```python
from build123d import *

# Parameters (mm, degrees)
SKETCH_R        = 14.1
SKETCH_R_2      = 1
PAD_DEPTH       = 38
SKETCH001_R     = 1.5
POCKET_DEPTH    = 3
SKETCH002_W     = 20
SKETCH002_H     = 2.5
SKETCH002_W_2   = 18
POCKET001_DEPTH = 34.001


with BuildPart() as part:
    # Sketch → Pad (new body)
    with BuildSketch(Plane.XY):
        Polygon((16, -16), (16, 16), (16, 18), (-16, 18), (-16, 16), (-16, -16), align=None)
        Circle(SKETCH_R, mode=Mode.SUBTRACT)
        with Locations((-12, 12)):
            Circle(SKETCH_R_2, mode=Mode.SUBTRACT)
        with Locations((12, 12)):
            Circle(SKETCH_R_2, mode=Mode.SUBTRACT)
        with Locations((12, -12)):
            Circle(SKETCH_R_2, mode=Mode.SUBTRACT)
        with Locations((-12, -12)):
            Circle(SKETCH_R_2, mode=Mode.SUBTRACT)
    extrude(amount=PAD_DEPTH)

    # Sketch001 (on Face5 of Pad) → Pocket (cut)
    with BuildSketch(Plane(origin=(0, 18, 0), x_dir=(-1, 0, 0), z_dir=(0, 1, 0))):
        with Locations((-12, 31)):
            Circle(SKETCH001_R)
        with Locations((12, 31)):
            Circle(SKETCH001_R)
        with Locations((12, 7)):
            Circle(SKETCH001_R)
        with Locations((-12, 7)):
            Circle(SKETCH001_R)
    extrude(amount=-POCKET_DEPTH, mode=Mode.SUBTRACT)

    # Sketch002 (on Face6 of Pocket) → Pocket001 (cut, through all)
    with BuildSketch(Plane(origin=(0, 18, 0), x_dir=(-1, 0, 0), z_dir=(0, 1, 0))):
        with Locations((0, 27.125)):
            Rectangle(SKETCH002_W, SKETCH002_H)
        with Locations((0, 23.0625)):
            Rectangle(SKETCH002_W, SKETCH002_H)
        with Locations((0, 19)):
            Rectangle(SKETCH002_W, SKETCH002_H)
        with Locations((0, 14.9375)):
            Rectangle(SKETCH002_W, SKETCH002_H)
        with Locations((0, 10.875)):
            Rectangle(SKETCH002_W, SKETCH002_H)
        with Locations((0, 6.8125)):
            Rectangle(SKETCH002_W_2, SKETCH002_H)
        with Locations((0, 31.1875)):
            Rectangle(SKETCH002_W_2, SKETCH002_H)
        with Locations((0, 2.75)):
            Rectangle(SKETCH002_W, SKETCH002_H)
        with Locations((0, 35.25)):
            Rectangle(SKETCH002_W, SKETCH002_H)
    extrude(amount=-POCKET001_DEPTH, mode=Mode.SUBTRACT)


solid = part.part
```
Can you work these out from the model? Positions are in its coordinate system, mm. A direction names the side the tool comes from. Round coordinates to 2 decimals unless told otherwise and drop trailing zeros. Loops run counter-clockwise (first coordinate to the right, second up) from the corner with the lowest first, then second, coordinate; pieces in that order, holes last.
Item 1: If we mould it in two halves opening along Z, with no side actions, what happens to faces 4 (the cylindrical face through (11.2, 11.4, 18.7)), 5 (the cylindrical face through (-10.89, 16.52, 32.01)), 6 (the flat face through (-7, 13, 38)), 7 (the flat face through (-7, 13, 0))? For each: +Z half, -Z half, draft (parallel to the pull), parting line (faces both ways), or undercut.
Item 2: Suppose I cut it at B-B, the plane x = 12.5. Write out the boundary of the cut face in (y, z), then the cut area to 3 significant figures.
Item 3: Will these pins go through, and if not, where does the flat tip stop? pin 1 Ø1.5 at (x, z) = (12, 6.5) entering from +Y; pin 2 Ø1.5 at (x, y) = (4, -12.5) entering from +Z.
Item 4: Which directions (+Z, -Z, +X, -X, +Y, -Y) give clear straight access to the entire face, cutting with the end or side of a thin tool? Please do faces 1 (the cylindrical face through (11, -12, 19)), 2 (the flat face through (-12, 15, 7)), 3 (the flat face through (0.1, -14.3, 34)).
Item 5: Please list where these lines run through material, in increasing order: L1, parallel to Z at x = 12, y = 16; L2, parallel to Y at x = 12, z = 24; L3, parallel to Y at x = -12, z = 30.
Item 6: Suppose I cut it at D-D, the plane z = 17. Write out the boundary of the cut face in (x, y), then the cut area to 3 significant figures.
Item 7: Suppose I cut it at A-A, the plane z = 31. Write out the boundary of the cut face in (x, y), then the cut area to 3 significant figures.
Item 8: Suppose I cut it at C-C, the plane y = -5. Write out the boundary of the cut face in (x, z), then the cut area to 3 significant figures.
Reported:
1. face 4: draft
1. face 5: undercut
1. face 6: +Z half
1. face 7: -Z half
2. outline: (-16, 0) - (-12.87, 0) - (-12.87, 38) - (-16, 38) - close; (-11.13, 0) - (-6.52, 0) - (-6.52, 38) - (-11.13, 38) - close; (6.52, 0) - (11.13, 0) - (11.13, 38) - (6.52, 38) - close; (12.87, 0) - (18, 0) - (18, 5.59) - (15, 5.59) - (15, 8.41) - (18, 8.41) - (18, 29.59) - (15, 29.59) - (15, 32.41) - (18, 32.41) - (18, 38) - (12.87, 38) - close
2. area: 648 mm2
3. pin 1: stops at y = 15
3. pin 2: passes through
4. face 1: +Z, -Z
4. face 2: +Y
4. face 3: +Y, -Y
5. L1: z = 0 to 5.5, 8.5 to 29.5, 32.5 to 38
5. L2: y = -16 to -13, -11 to -7.4, 7.4 to 11, 13 to 18
5. L3: y = -16 to -13, -11 to -7.4, 7.4 to 11, 13 to 15
6. outline: (-16, -16) - (16, -16) - (16, 18) - (-16, 18) - close; hole circle Ø28.2 at (0, 0); hole circle Ø2 at (-12, -12); hole circle Ø2 at (-12, 12); hole circle Ø2 at (12, -12); hole circle Ø2 at (12, 12)
6. area: 451 mm2
7. outline: (-16, -16) - (-9, -16) - (-9, -10.85) arc R14.1 cw to (-9, 10.85) - (-9, 18) - (-10.5, 18) - (-10.5, 15) - (-13.5, 15) - (-13.5, 18) - (-16, 18) - close; (9, -16) - (16, -16) - (16, 18) - (13.5, 18) - (13.5, 15) - (10.5, 15) - (10.5, 18) - (9, 18) - (9, 10.85) arc R14.1 cw to (9, -10.85) - close; hole circle Ø2 at (-12, -12); hole circle Ø2 at (-12, 12); hole circle Ø2 at (12, -12); hole circle Ø2 at (12, 12)
7. area: 291 mm2
8. outline: (-16, 0) - (-13.18, 0) - (-13.18, 38) - (-16, 38) - close; (13.18, 0) - (16, 0) - (16, 38) - (13.18, 38) - close
8. area: 214 mm2
